Source: three-view drawing plus pictorial views. Frame: mm from the lowest corner of the part. A direction names the side the tool comes from. Give positions to 0.01 mm unless a question says otherwise; leave off trailing zeros. Loops run counter-clockwise (first coordinate to the right, second up) from the corner with the lowest first, then second, coordinate; pieces in that order, holes last.
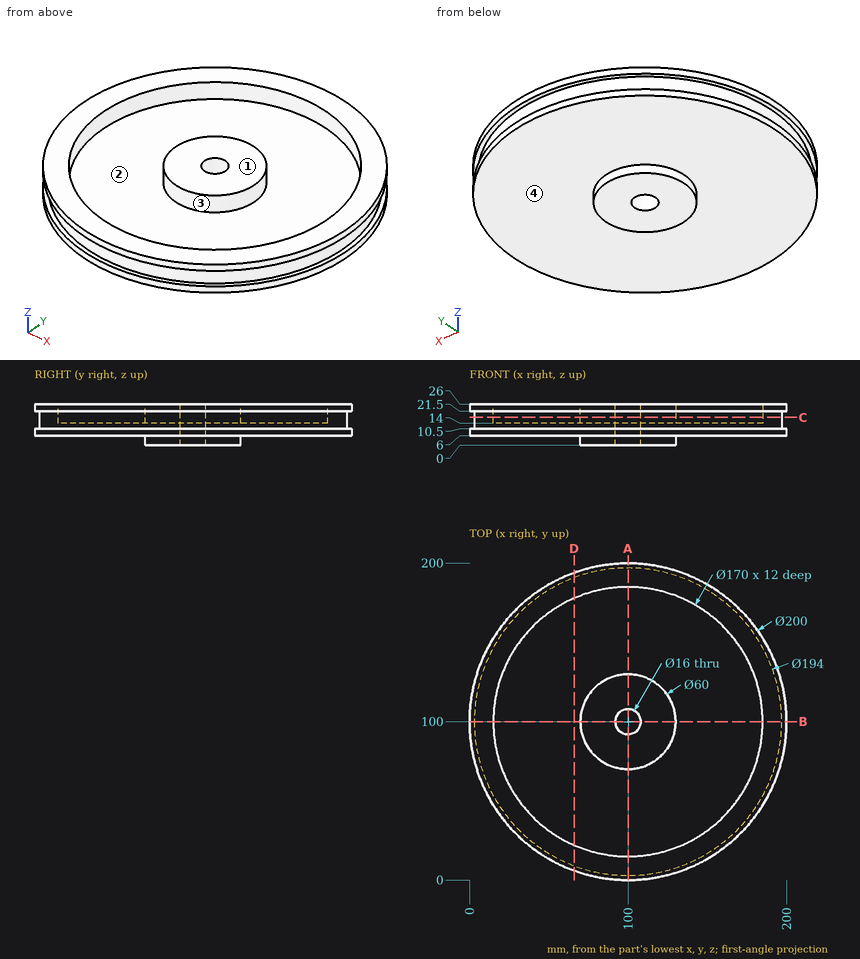
Q1. Material intervals for probe 1 along Y at (x, z) = (100, 19); probe 2 along Y at (x, z) = (100, 12); probe 3 along Z at (x, y) = (138, 120), sorted ascending.
Q2. Mould query, pull axis Y, two halves, no side actions, for the marked faces 3 and 4. Classes: +Y half, -Y half, draft (parallel to the pull), parting line (faces both ways), or undercut.
Q3. Section query A-A, the plane x = 100. Return loops of the section in (y, z).
Q4. Reachability of the marked faces 1 and 2 from +Z, -Z, +X, -X, +Y, -Y: full face, straight path, thin tool, end or side. Return the list, or none.
Q5. Section query C-C, the plane z = 17.5. Return loops of the section in (x, y), and give its area (3 significant figures).
Q6. Section query D-D, the plane x = 66. Return loops of the section in (y, z).
Q7. Pin query (flat end, axial travel): pin 1 Ø4 at (x, z) = (78, 17) entering from +Y; pin 2 Ø1 at (x, z) = (174.5, 12) entering from -Y; pin 3 Ø6 at (y, z) = (85.5, 21.5) entering from -X. Return the tip coordinate at first contact, or that it passes through.
Resolved:
1. probe 1: y = 3 to 15, 70 to 92, 108 to 130, 185 to 197
1. probe 2: y = 3 to 92, 108 to 197
1. probe 3: z = 6 to 14
2. face 3: undercut
2. face 4: draft
3. outline: (0, 6) - (70, 6) - (70, 0) - (92, 0) - (92, 26) - (70, 26) - (70, 14) - (15, 14) - (15, 26) - (0, 26) - (0, 21.5) - (3, 21.5) - (3, 10.5) - (0, 10.5) - close; (108, 0) - (130, 0) - (130, 6) - (200, 6) - (200, 10.5) - (197, 10.5) - (197, 21.5) - (200, 21.5) - (200, 26) - (185, 26) - (185, 14) - (130, 14) - (130, 26) - (108, 26) - close
4. face 1: +Z, +X, -X, +Y, -Y
4. face 2: +Z
5. outline: circle Ø194 at (100, 100); circle Ø60 at (100, 100); hole circle Ø170 at (100, 100); hole circle Ø16 at (100, 100)
5. area: 9,490 mm2
6. outline: (5.96, 6) - (194.04, 6) - (194.04, 10.5) - (190.85, 10.5) - (190.85, 21.5) - (194.04, 21.5) - (194.04, 26) - (177.9, 26) - (177.9, 14) - (22.1, 14) - (22.1, 26) - (5.96, 26) - (5.96, 21.5) - (9.15, 21.5) - (9.15, 10.5) - (5.96, 10.5) - close
7. pin 1: stops at y = 194.92
7. pin 2: stops at y = 37.29
7. pin 3: stops at x = 0.66
